from build123d import *

# Parameters (mm, degrees)
BOSS_EXTRUDE1_DEPTH = 55
SKETCH2_R           = 1.25
CUT_EXTRUDE1_DEPTH  = 12
CUT_EXTRUDE2_START  = -12
SKETCH3_R           = 1.25
CUT_EXTRUDE2_DEPTH  = 12


with BuildPart() as part:
    # Sketch1 → Boss-Extrude1 (new body)
    with BuildSketch(Plane(origin=(0, 0, 0), x_dir=(1, 0, 0), z_dir=(0, 1, 0))):
        Polygon((0, 3.5), (-3.5, 3.5), (-3.5, -3.5), (3.5, -3.5), (3.5, 3.5), align=None)
    extrude(amount=BOSS_EXTRUDE1_DEPTH)

    # Sketch2 → Cut-Extrude1 (cut)
    with BuildSketch(Plane(origin=(0, 55, 0), x_dir=(1, 0, 0), z_dir=(0, 1, 0))):
        with Locations(Location((0, 0, 0), (0, 0, 270))):
            Circle(SKETCH2_R)
    extrude(amount=-CUT_EXTRUDE1_DEPTH, mode=Mode.SUBTRACT)

    # Sketch3 → Cut-Extrude2 (cut)
    with BuildSketch(Plane.XZ.offset(CUT_EXTRUDE2_START)):
        with Locations(Location((0, 0, 0), (0, 0, 90))):
            Circle(SKETCH3_R)
    extrude(amount=CUT_EXTRUDE2_DEPTH, mode=Mode.SUBTRACT)


solid = part.part
Input: part model. Units: mm. Frame: model coordinates. A direction names the side the tool comes from. Coordinates: 2 decimals unless noted, no trailing zeros. Loops run counter-clockwise (first coordinate to the right, second up) from the corner with the lowest first, then second, coordinate; pieces in that order, holes last. Notation, with made-up numbers: (-28, -8) -> (-10, -8) arc R26 cw to (-10, 7) -> close; hole circle Ø5 at (68, 83). An arc over 180 degrees is marked (long way). Write each question's results on one line, items separated by ' | '. Start each with the question number.
Q1. Reachability of faces 1 (the flat face through (0, 43, 0)), 2 (the flat face through (0, 12, 0)), 3 (the flat face through (-2, 55, 0)) from +Z, -Z, +X, -X, +Y, -Y: full face, straight path, thin tool, end or side. Return the list, or none.
Q2. Pull-direction query (Z, two-part tool) for faces 4 (the flat face through (-2, 0, 0)), 5 (the cylindrical face through (1.22, 6.08, -0.27)), 6 (the flat face through (0, 27, -3.5)); classes: released by +Z, released by -Z, zero draft, split by the parting line, or undercut.
Q3. Pin query (flat end, axial travel): pin 1 (1.5 mm diameter, centred on x = 0, z = 0, fed in from +Y); pin 2 (2 mm diameter, centred on x = 0, z = 0, fed in from -Y). Return the tip coordinate at first contact, or that it passes through.
Q4. Section B-B, the plane x = -0.75. Return the cut outline in (y, z).
Q5. Section A-A, the plane z = 0. Return the cut outline in (x, y).
Q6. Ray query, line 1 (X direction, y = 7, z = 0); line 2 (Y direction, x = 0.25, z = 0.5). Return the intervals inside material, ascending. Write a range as from..to.
Found:
1) face 1: +Y | face 2: -Y | face 3: +Z, -Z, +X, -X, +Y
2) face 4: zero draft | face 5: undercut | face 6: released by -Z
3) pin 1: y = 43 | pin 2: y = 12
4) outline: (0, -3.5) -> (55, -3.5) -> (55, -1) -> (43, -1) -> (43, 1) -> (55, 1) -> (55, 3.5) -> (0, 3.5) -> (0, 1) -> (12, 1) -> (12, -1) -> (0, -1) -> close
5) outline: (-3.5, 0) -> (-1.25, 0) -> (-1.25, 12) -> (1.25, 12) -> (1.25, 0) -> (3.5, 0) -> (3.5, 55) -> (1.25, 55) -> (1.25, 43) -> (-1.25, 43) -> (-1.25, 55) -> (-3.5, 55) -> close
6) line 1: -3.5..-1.25, 1.25..3.5 | line 2: 12..43
